Job drawing, mm, ordinate dimensions from the low corner. One solid piece. A direction names the side the tool comes from. Give positions to 0.01 mm unless a question says otherwise; leave off trailing zeros. Loops run counter-clockwise (first coordinate to the right, second up) from the corner with the lowest first, then second, coordinate; pieces in that order, holes last. Notation, with made-up numbers: (20, 12) -> (77, 12) arc R19 ccw to (77, 38) -> close; hole circle Ø10 at (51, -24.75). An arc over 180 degrees is marked (long way). Answer as a JSON object with one key per item and string values. Group by question number.
Q1. Band-saw the part on C-C, the plane y = 37. Write the cut outline in (x, z).
Q2. Tool access for the marked faces 1 and 2: list every direction of +Z, -Z, +X, -X, +Y, -Y with a clear straight run to the whole face (end or side of a thin tool).
Q3. Wall check: probe 1 along Y at (x, z) = (2.25, 5.75); probe 2 along Y at (x, z) = (4.5, 7); probe 3 along X at (y, z) = (15.5, 3.75). Give the ranges that are in metal, low to high. Write a range as from..to.
Q4. Band-saw the part on B-B, the plane x = 4. Write the cut outline in (y, z), plus the area to 3 significant figures.
Q5. Band-saw the part on A-A, the plane z = 4. Write the cut outline in (x, y), plus the area to 3 significant figures.
Q6. Drop flat-ended pins along their axis: pin 1 (2 mm diameter, centred on x = 6, z = 3, fed in from -Y); pin 2 (1 mm diameter, centred on y = 23, z = 5, fed in from -X); pin 3 (3 mm diameter, centred on x = 1, y = 53.5, fed in from -Z). Give the stop position or say it passes through.
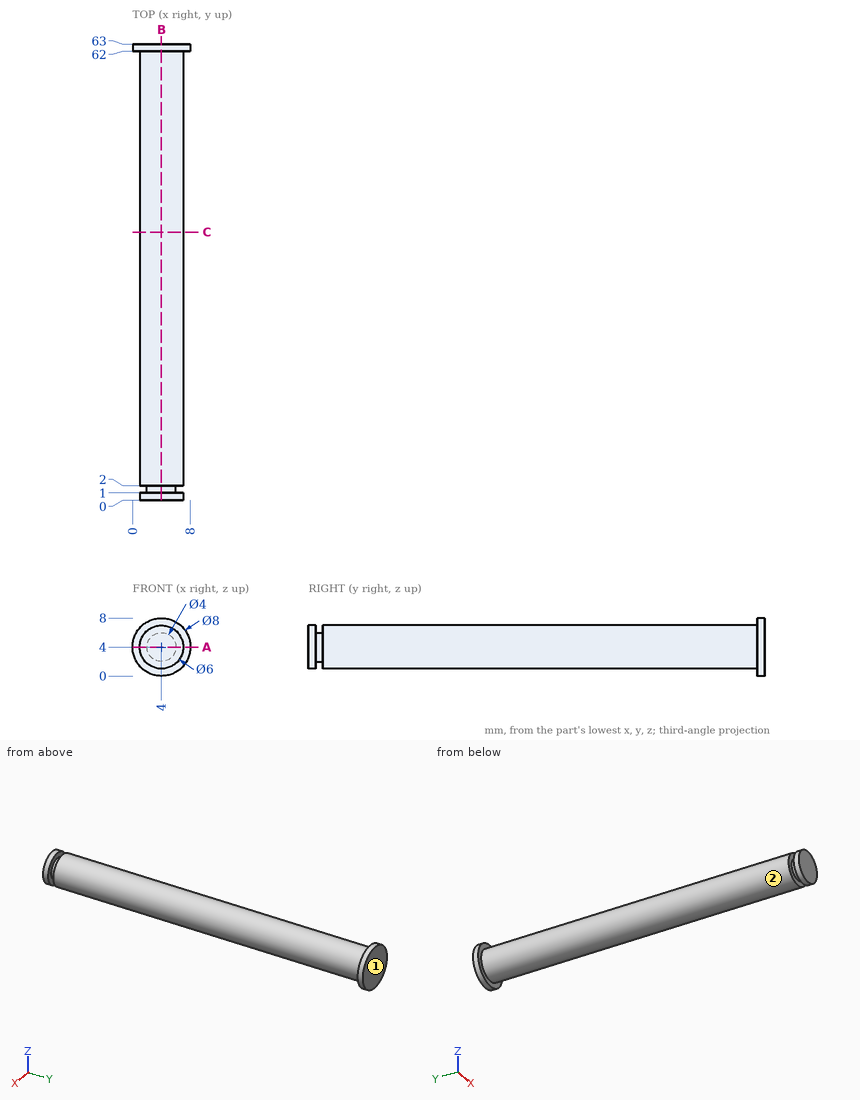
Worked answers:
{
 "1": {"outline": "circle Ø6 at (4, 4)"},
 "2": {"face 1": "+Z, -Z, +X, -X, +Y", "face 2": "-Y"},
 "3": {"probe 1": "0..1, 2..63", "probe 2": "62..63", "probe 3": "1.01..6.99"},
 "4": {"outline": "(0, 1) -> (1, 1) -> (1, 2) -> (2, 2) -> (2, 1) -> (62, 1) -> (62, 0) -> (63, 0) -> (63, 8) -> (62, 8) -> (62, 7) -> (2, 7) -> (2, 6) -> (1, 6) -> (1, 7) -> (0, 7) -> close", "area": "378 mm2"},
 "5": {"outline": "(0, 62) -> (1, 62) -> (1, 2) -> (2, 2) -> (2, 1) -> (1, 1) -> (1, 0) -> (7, 0) -> (7, 1) -> (6, 1) -> (6, 2) -> (7, 2) -> (7, 62) -> (8, 62) -> (8, 63) -> (0, 63) -> close", "area": "378 mm2"},
 "6": {"pin 1": "y = 0", "pin 2": "x = 1.04", "pin 3": "z = 1.4"}
}
